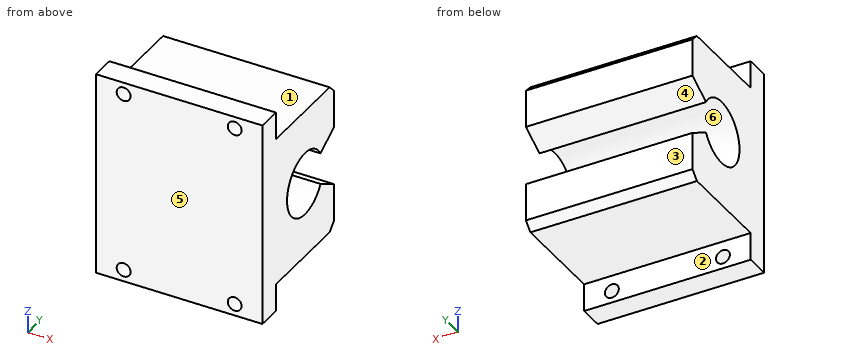
```python
from build123d import *

# Parameters (mm, degrees)
SKETCH1_R            = 12.7
BASE_EXTRUDE_DEPTH   = 66.675
SKETCH2_R            = 2.778125
CUT_EXTRUDE1_DEPTH   = 89.61606443
LPATTERN1_COUNT      = 2
LPATTERN1_PITCH      = 44.45
LPATTERN1_COUNT_DIR2 = 2
LPATTERN1_PITCH_DIR2 = 73.025
CUT_EXTRUDE2_DEPTH   = 94.433512457
CHAMFER1_SIZE        = 3.175


with BuildPart() as part:
    # Sketch1 → Base-Extrude (new body)
    with BuildSketch(Plane(origin=(0, 0, 0), x_dir=(0, 0, -1), z_dir=(1, 0, 0))):
        Polygon((-41.275, 0), (41.275, 0), (41.275, 9.525), (30.1625, 9.525), (30.1625, 50.8), (-30.1625, 50.8), (-30.1625, 9.525), (-41.275, 9.525), align=None)
        with Locations((0, 30.1625)):
            Circle(SKETCH1_R, mode=Mode.SUBTRACT)
    extrude(amount=BASE_EXTRUDE_DEPTH)

    # Sketch2 → Cut-Extrude1 (cut, through all)
    with BuildSketch(Plane(origin=(0, 9.525, 0), x_dir=(-1, 0, 0), z_dir=(0, 1, 0))):
        with Locations(Location((-55.5625, 36.5125, 0), (0, 0, 90))):
            Circle(SKETCH2_R)
    cut_extrude1 = extrude(amount=-CUT_EXTRUDE1_DEPTH, mode=Mode.SUBTRACT)

    # LPattern1: Cut-Extrude1 2 × 2
    with Locations(*[(-i * LPATTERN1_PITCH, 0, -j * LPATTERN1_PITCH_DIR2) for i in range(LPATTERN1_COUNT) for j in range(LPATTERN1_COUNT_DIR2) if (i, j) != (0, 0)]):
        add(cut_extrude1, mode=Mode.SUBTRACT)

    # Sketch3 → Cut-Extrude2 (cut, through all)
    with BuildSketch(Plane(origin=(66.675, 0, 0), x_dir=(0, 0, -1), z_dir=(1, 0, 0))):
        Polygon((11.91506618, 50.8), (-11.91506618, 50.8), (0, 30.1625), align=None)
    extrude(amount=-CUT_EXTRUDE2_DEPTH, mode=Mode.SUBTRACT)

    # Chamfer1
    chamfer1_edges = [part.edges().sort_by_distance(p)[0] for p in [
        (33.3375, 50.8, 30.1625),
        (33.3375, 50.8, -30.1625),
    ]]
    chamfer(chamfer1_edges, length=CHAMFER1_SIZE)


solid = part.part
```
Work out the finished part from the listing and answer in its coordinate system (mm). Face numbers are marked on the shaded views. A direction names the side the tool comes from. Round coordinates to 2 decimals unless told otherwise and drop trailing zeros. Write each loop counter-clockwise with the first axis right and the second up, starting at its lowest first coordinate (ties: lowest second). Pieces come first, ordered by that corner, then holes.
1) A cutting plane is placed at A-A on y = 33. Determine the outline of the cut face in (x, z) (1 decimal).
2) A cutting plane is placed at D-D on y = 7.5. Determine the outline of the cut face in (x, z) (1 decimal).
3) Consider probe 1 along Z at (x, y) = (54, 5) (3 decimals); probe 2 along Z at (x, y) = (13, 31); probe 3 along Z at (x, y) = (39.5, 20). Determine where each line is inside the solid, lowest interval first.
4) A cutting plane is placed at C-C on z = 9.5. Determine the outline of the cut face in (x, y) (3 decimals), and give its area (3 significant figures).
5) Which of the six approach directions +Z, -Z, +X, -X, +Y, -Y give full straight-line access (tool end or side, diameter ignored) to the marked faces 1, 2 and 3?
6) Flat-ended cylindrical pins translate along their axes: P1, Ø1, axis at y = 10.5, z = -13, coming from the -X side; P2, Ø3.5, axis at x = 55.56, z = -36.51, coming from the +Y side; P3, Ø9, axis at x = 23, z = 37.5, coming from the +Y side (3 decimals); P4, Ø4, axis at x = 46, z = -31, coming from the +Y side. Find the tip coordinate at first contact, or state that the pin passes through.
7) A cutting plane is placed at B-B on x = 54.5. Give the number of separate pieces and of enclosed holes in the cut face, and give its area (3 significant figures).
8) Determine the mould class of the marked faces 4, 5 and 6 for opening direction Y: pulls with the +Y half, pulls with the -Y half, needs draft (parallel to the pull), parting line crosses it, or undercut.
Entries:
1. outline: (0, -30.2) - (66.7, -30.2) - (66.7, -12.4) - (0, -12.4) - close; (0, 12.4) - (66.7, 12.4) - (66.7, 30.2) - (0, 30.2) - close
2. outline: (0, -41.3) - (66.7, -41.3) - (66.7, 41.3) - (0, 41.3) - close; hole circle Ø5.6 at (11.1, -36.5); hole circle Ø5.6 at (11.1, 36.5); hole circle Ø5.6 at (55.6, -36.5); hole circle Ø5.6 at (55.6, 36.5)
3. probe 1: z = -41.275 to -38.81, -34.215 to 34.215, 38.81 to 41.275
3. probe 2: z = -30.16 to -12.67, 12.67 to 30.16
3. probe 3: z = -30.16 to -7.62, 7.62 to 30.16
4. outline: (0, 0) - (66.675, 0) - (66.675, 21.734) - (0, 21.734) - close; (0, 38.591) - (66.675, 38.591) - (66.675, 46.617) - (0, 46.617) - close
4. area: 1,980 mm2
5. face 1: +Z, +X, -X, +Y
5. face 2: -Z, +X, -X, +Y
5. face 3: +Z, -Z, +X, -X, +Y
6. P1: stops at x = 0
6. P2: passes through
6. P3: stops at y = 9.525
6. P4: stops at y = 48.79
7. separate pieces: 3
7. enclosed holes: 0
7. area: 2,500 mm2
8. face 4: pulls with the +Y half
8. face 5: pulls with the -Y half
8. face 6: undercut
